Check sheet for the modelled part. Datum: model origin and axes. Units: mm. Round coordinates to 2 decimals unless told otherwise and drop trailing zeros. Order: outer loops, then holes, each group sorted by start corner. A loop starts at its lowest first (then second) coordinate and runs counter-clockwise, first axis right, second up. Notation, with made-up numbers: (82, 12.5) -> (101, 12.5) arc R29 cw to (101, 49.5) -> close; hole circle Ø5 at (29, 36.5). An arc over 180 degrees is marked (long way). Answer in a Markdown table with one row per item. Add a question column.
1. Sectioned sample at D-D, the plane x = 240. Record the boundary of the cut face in (y, z), then the cut area to 3 significant figures.
2. Depth check by flat-ended pin: P1, Ø3, axis at x = 163, z = 1.5, coming from the +Y side; P2, Ø5.5, axis at x = 240, y = -55, coming from the +Z side. Enter the tip coordinate at first touch or a pass-through.
3. Sectioned sample at B-B, the plane z = 2.95. Record the boundary of the cut face in (x, y).
4. Sectioned sample at C-C, the plane y = -55. Record the boundary of the cut face in (x, z), then the cut area to 3 significant figures.
5. Sectioned sample at A-A, the plane y = -5. Record the boundary of the cut face in (x, z), then the cut area to 3 significant figures.
6. Material ranges on L1, parallel to Y at x = 240, z = 2.15; L2, parallel to X at y = -9, z = 2.3; L3, parallel to X at y = -7, z = 4.45, recorded low to high. Write a range as from..to.
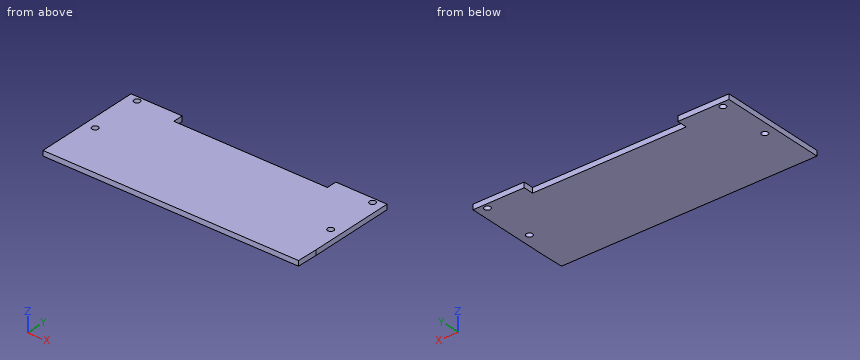
```python
from build123d import *

# Parameters (mm, degrees)
ESQUISSE1_W             = 250
ESQUISSE1_H             = 85
ESQUISSE1_R             = 3
BOSS_EXTRU_1_DEPTH      = 5
BOSS_EXTRU_2_DEPTH      = 5
ESQUISSE3_W             = 150
ESQUISSE3_H             = 10
ENL_V_MAT_EXTRU_1_DEPTH = 10


with BuildPart() as part:
    # Esquisse1 → Boss.-Extru.1 (new body)
    with BuildSketch(Plane.XY):
        with Locations((125, -42.5)):
            Rectangle(ESQUISSE1_W, ESQUISSE1_H)
        with Locations((10, -5)):
            Circle(ESQUISSE1_R, mode=Mode.SUBTRACT)
        with Locations((10, -55)):
            Circle(ESQUISSE1_R, mode=Mode.SUBTRACT)
        with Locations(Location((240, -55, 0), (0, 0, 180))):
            Circle(ESQUISSE1_R, mode=Mode.SUBTRACT)
        with Locations(Location((240, -5, 0), (0, 0, 180))):
            Circle(ESQUISSE1_R, mode=Mode.SUBTRACT)
    extrude(amount=BOSS_EXTRU_1_DEPTH)

    # Esquisse2 → Boss.-Extru.2 (add)
    with BuildSketch(Plane.XY.offset(5)):
        Polygon((0, -85), (0, -105), (249.491359447, -105), (250, -85), align=None)
    extrude(amount=-BOSS_EXTRU_2_DEPTH)

    # Esquisse3 → Enlèv. mat.-Extru.1 (cut)
    with BuildSketch(Plane(origin=(0, 0, 0), x_dir=(-1, 0, 0), z_dir=(0, 0, -1))):
        with Locations((-125, -5)):
            Rectangle(ESQUISSE3_W, ESQUISSE3_H)
    extrude(amount=-ENL_V_MAT_EXTRU_1_DEPTH, mode=Mode.SUBTRACT)


solid = part.part
```
Answer key:
| question | item | result |
|---|---|---|
| 1 | outline | (-105, 0) -> (-58, 0) -> (-58, 5) -> (-105, 5) -> close; (-52, 0) -> (-8, 0) -> (-8, 5) -> (-52, 5) -> close; (-2, 0) -> (0, 0) -> (0, 5) -> (-2, 5) -> close |
| 1 | area | 465 mm² |
| 2 | P1 | stops at y = -10 |
| 2 | P2 | passes through |
| 3 | outline | (0, -105) -> (249.49, -105) -> (250, -85) -> (250, 0) -> (200, 0) -> (200, -10) -> (50, -10) -> (50, 0) -> (0, 0) -> close; hole circle Ø6 at (10, -55); hole circle Ø6 at (10, -5); hole circle Ø6 at (240, -55); hole circle Ø6 at (240, -5) |
| 4 | outline | (0, 0) -> (7, 0) -> (7, 5) -> (0, 5) -> close; (13, 0) -> (237, 0) -> (237, 5) -> (13, 5) -> close; (243, 0) -> (250, 0) -> (250, 5) -> (243, 5) -> close |
| 4 | area | 1,190 mm² |
| 5 | outline | (0, 0) -> (7, 0) -> (7, 5) -> (0, 5) -> close; (13, 0) -> (50, 0) -> (50, 5) -> (13, 5) -> close; (200, 0) -> (237, 0) -> (237, 5) -> (200, 5) -> close; (243, 0) -> (250, 0) -> (250, 5) -> (243, 5) -> close |
| 5 | area | 440 mm² |
| 6 | L1 | y = -105..-58, -52..-8, -2..0 |
| 6 | L2 | x = 0..50, 200..250 |
| 6 | L3 | x = 0..7.76, 12.24..50, 200..237.76, 242.24..250 |
